Geometry check sheet. Reference: drawing and pictorial views, mm from the part's lowest x, y, z. Coordinates: 2 decimals unless noted, no trailing zeros. Write each loop counter-clockwise with the first axis right and the second up, starting at its lowest first coordinate (ties: lowest second). Pieces come first, ordered by that corner, then holes. Notation, with made-up numbers: (52, 12.25) -> (68, 12.25) arc R14 ccw to (68, 20.25) -> close; hole circle Ø1 at (59, 22.5). An arc over 180 degrees is marked (long way). Put each result on its own line as item: value.
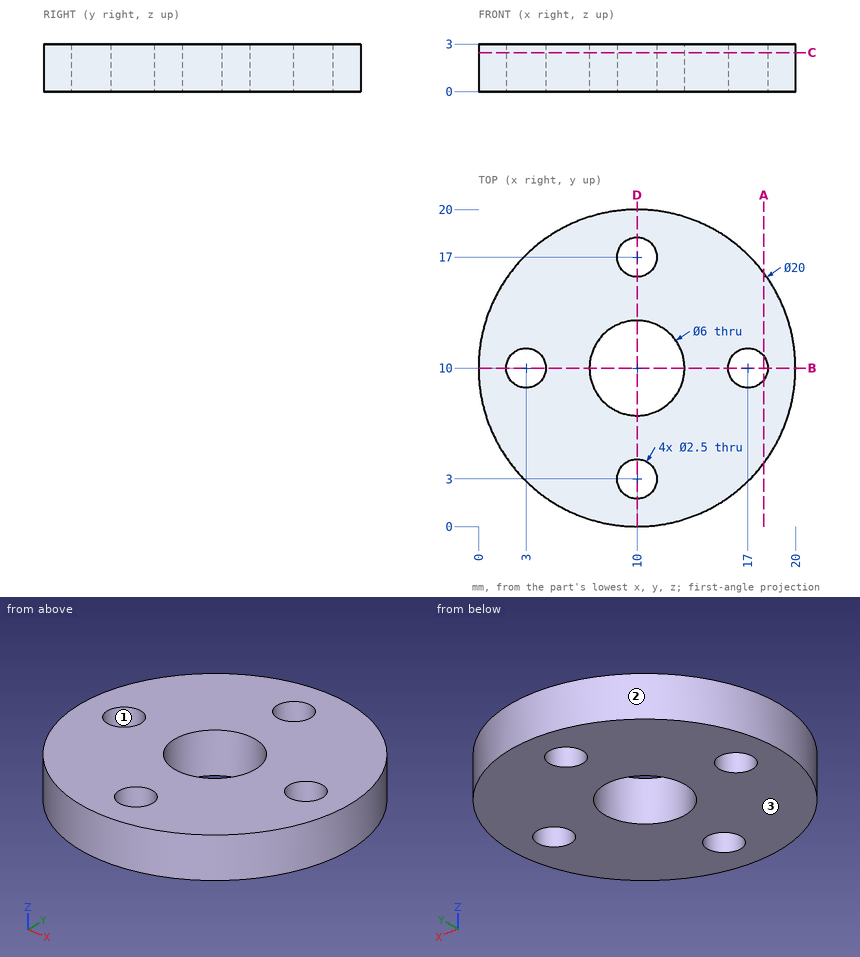
Q1. Depth check by flat-ended pin: P1, Ø1.5, axis at y = 8, z = 2, coming from the +X side; P2, Ø1.5, axis at x = 9, z = 1.5, coming from the +Y side. Enter the tip coordinate at first touch or a pass-through.
Recorded:
P1: stops at x = 19.92
P2: stops at y = 20
Q2. Mould release check, pull along X, two halves, no side actions. Record for the marked faces 1, 2 and 3: released by +X, released by -X, zero draft, split by the parting line, or undercut.
Recorded:
face 1: undercut
face 2: split by the parting line
face 3: zero draft
Q3. Material ranges on line 1 along Y through (x, z) = (10, 1.55); line 2 along Y through (x, z) = (8.5, 0.2); line 3 along Y through (x, z) = (3, 0.35), recorded low to high.
Recorded:
line 1: y = 0 to 1.75, 4.25 to 7, 13 to 15.75, 18.25 to 20
line 2: y = 0.11 to 7.4, 12.6 to 19.89
line 3: y = 2.86 to 8.75, 11.25 to 17.14
Q4. Cross-section at B-B (y = 10). Record the cut outline in (x, z), plus the area to 3 significant figures.
Recorded:
outline: (0, 0) -> (1.75, 0) -> (1.75, 3) -> (0, 3) -> close; (4.25, 0) -> (7, 0) -> (7, 3) -> (4.25, 3) -> close; (13, 0) -> (15.75, 0) -> (15.75, 3) -> (13, 3) -> close; (18.25, 0) -> (20, 0) -> (20, 3) -> (18.25, 3) -> close
area: 27.0 mm2
Q5. Cross-section at C-C (z = 2.45). Record the cut outline in (x, y).
Recorded:
outline: circle Ø20 at (10, 10); hole circle Ø2.5 at (3, 10); hole circle Ø6 at (10, 10); hole circle Ø2.5 at (10, 3); hole circle Ø2.5 at (10, 17); hole circle Ø2.5 at (17, 10)
Q6. Cross-section at A-A (x = 18). Record the cut outline in (y, z).
Recorded:
outline: (4, 0) -> (9.25, 0) -> (9.25, 3) -> (4, 3) -> close; (10.75, 0) -> (16, 0) -> (16, 3) -> (10.75, 3) -> close
